Input: part model. Units: mm. Frame: model coordinates. Face numbers are marked on the shaded views. Round coordinates to 2 decimals unless told otherwise and drop trailing zeros. Loops run counter-clockwise (first coordinate to the right, second up) from the corner with the lowest first, then second, coordinate; pieces in that order, holes last. Notation, with made-up numbers: (71, -11) - (84, -11) arc R17 cw to (84, 1) - close; hole circle Ø11 at (-27.5, -19.75). An arc over 180 degrees is marked (long way). One line per question, with ' | ' between items. Start each with the question number.
Item 1: Section B-B, the plane x = 22. Return loops of the section in (y, z), plus the area to 3 significant figures.
Item 2: Section D-D, the plane y = 30.5. Return loops of the section in (x, z), plus the area to 3 significant figures.
Item 3: Material intervals for line 1 along Y through (x, z) = (20, -15); line 2 along X through (y, z) = (31.5, -15); line 3 along Y through (x, z) = (21.5, -42), sorted ascending.
Item 4: First-contact query: pin 1 (12 mm diameter, centred on x = 11, z = -30.5, fed in from -Y); pin 2 (1.3 mm diameter, centred on x = 13.5, z = -23, fed in from +Y); pin 3 (3 mm diameter, centred on x = 1.5, y = 9.5, fed in from -Z); pin 4 (10 mm diameter, centred on y = 4, z = -32.5, fed in from -X). Flat tips, straight axial feed; report the tip coordinate or a pass-through.
Item 5: Section A-A, the plane z = -22. Return loops of the section in (x, y), plus the area to 3 significant figures.
Item 6: Draft query along Y for the marked faces 1, 2 and 3. Return one class per face: pulls with the +Y half, pulls with the -Y half, needs draft (parallel to the pull), parting line crosses it, or undercut.
Item 7: Section C-C, the plane z = -5.5. Return loops of the section in (x, y).
```python
from build123d import *

# Parameters (mm, degrees)
BOSS_EXTRUDE1_DEPTH      = 2.54
BOSS_EXTRUDE2_DEPTH      = 2.54
BOSS_EXTRUDE2_DEPTH_BACK = 12.7
SKETCH3_R                = 1.778
SKETCH4_R                = 34.29
BOSS_EXTRUDE3_DEPTH      = 10.16
BOSS_EXTRUDE4_DEPTH      = 2.54
BOSS_EXTRUDE5_DEPTH      = 10.16
BOSS_EXTRUDE5_DEPTH_BACK = 5.08
SKETCH6_R                = 1.778
SKETCH7_R                = 33.02
CUT_EXTRUDE1_DEPTH       = 7.62
SKETCH9_R                = 2.54
BOSS_EXTRUDE6_DEPTH      = 1.27
SKETCH10_R               = 1.27
BOSS_EXTRUDE7_DEPTH      = 20.32
CUT_EXTRUDE2_REACH       = 65.993
CUT_EXTRUDE3_REACH       = 65.993


with BuildPart() as part:
    # Sketch2 → Boss-Extrude1 (new body)
    with BuildSketch(Plane(origin=(0, 0, 0), x_dir=(0, 0, -1), z_dir=(1, 0, 0))):
        with BuildLine():
            Line((0, -1.778), (30.48, -1.778))
            ThreePointArc((30.48, -1.778), (32.258, 0), (30.48, 1.778))
            Line((30.48, 1.778), (0, 1.778))
            ThreePointArc((0, 1.778), (-1.778, 0), (0, -1.778))
        make_face()
    extrude(amount=BOSS_EXTRUDE1_DEPTH)

    # Sketch3 → Boss-Extrude2 (add, two sides: drawn at the far end of the back side and taken through both)
    with BuildSketch(Plane.ZY.offset(-BOSS_EXTRUDE2_DEPTH_BACK)):
        with Locations((-30.48, 0)):
            Circle(SKETCH3_R)
        Circle(SKETCH3_R)
    extrude(amount=BOSS_EXTRUDE2_DEPTH + BOSS_EXTRUDE2_DEPTH_BACK)

    # Sketch4 → Boss-Extrude3 (add)
    with BuildSketch(Plane(origin=(12.7, 0, 0), x_dir=(0, 0, -1), z_dir=(1, 0, 0))):
        with Locations((15.24, 0)):
            Circle(SKETCH4_R)
    extrude(amount=BOSS_EXTRUDE3_DEPTH)

    # Sketch5 → Boss-Extrude4 (add)
    with BuildSketch(Plane(origin=(0, 0, 0), x_dir=(0, 0, -1), z_dir=(1, 0, 0))):
        with BuildLine():
            Line((13.462, -19.05), (13.462, 19.05))
            ThreePointArc((13.462, 19.05), (15.24, 20.828), (17.018, 19.05))
            Line((17.018, 19.05), (17.018, -19.05))
            ThreePointArc((17.018, -19.05), (15.24, -20.828), (13.462, -19.05))
        make_face()
    extrude(amount=BOSS_EXTRUDE4_DEPTH)

    # Sketch6 → Boss-Extrude5 (add, two sides: drawn at the far end of the back side and taken through both)
    with BuildSketch(Plane(origin=(2.54, 0, 0), x_dir=(0, 0, -1), z_dir=(1, 0, 0)).offset(-BOSS_EXTRUDE5_DEPTH_BACK)):
        with Locations((15.24, -19.05)):
            Circle(SKETCH6_R)
        with Locations((15.24, 19.05)):
            Circle(SKETCH6_R)
    extrude(amount=BOSS_EXTRUDE5_DEPTH + BOSS_EXTRUDE5_DEPTH_BACK)

    # Sketch7 → Cut-Extrude1 (cut)
    with BuildSketch(Plane(origin=(22.86, 0, 0), x_dir=(0, 0, -1), z_dir=(1, 0, 0))):
        with Locations((15.24, 0)):
            Circle(SKETCH7_R)
    extrude(amount=-CUT_EXTRUDE1_DEPTH, mode=Mode.SUBTRACT)

    # Sketch9 → Boss-Extrude6 (add)
    with BuildSketch(Plane(origin=(15.24, 0, 0), x_dir=(0, 0, -1), z_dir=(1, 0, 0))):
        Circle(SKETCH9_R)
        with Locations((30.48, 0)):
            Circle(SKETCH9_R)
    extrude(amount=BOSS_EXTRUDE6_DEPTH)

    # Sketch10 → Boss-Extrude7 (add)
    with BuildSketch(Plane(origin=(16.51, 0, 0), x_dir=(0, 0, -1), z_dir=(1, 0, 0))):
        with Locations((30.48, 0)):
            Circle(SKETCH10_R)
        Circle(SKETCH10_R)
    extrude(amount=BOSS_EXTRUDE7_DEPTH)

    # Sketch11 → Cut-Extrude2 (cut, up to next)
    with BuildSketch(Plane(origin=(15.24, 0, 0), x_dir=(0, 0, -1), z_dir=(1, 0, 0)), mode=Mode.PRIVATE) as cut_extrude2_sk1:
        with BuildLine():
            Line((14.51, 5), (15.97, 5))
            ThreePointArc((15.97, 5), (16.868025612, 4.628025612), (17.24, 3.73))
            Line((17.24, 3.73), (17.24, -3.73))
            ThreePointArc((17.24, -3.73), (16.868025612, -4.628025612), (15.97, -5))
            Line((15.97, -5), (14.51, -5))
            ThreePointArc((14.51, -5), (13.611974388, -4.628025612), (13.24, -3.73))
            Line((13.24, -3.73), (13.24, 3.73))
            ThreePointArc((13.24, 3.73), (13.611974388, 4.628025612), (14.51, 5))
        make_face()
    cut_extrude2_tool1 = extrude(cut_extrude2_sk1.sketch, amount=-CUT_EXTRUDE2_REACH, mode=Mode.PRIVATE) & part.part
    add(cut_extrude2_tool1.solids().sort_by_distance((15.24, 0, -15.24))[0], mode=Mode.SUBTRACT)

    # Sketch15 → Cut-Extrude3 (cut, up to next)
    with BuildSketch(Plane(origin=(15.24, 0, 0), x_dir=(0, 0, -1), z_dir=(1, 0, 0)), mode=Mode.PRIVATE) as cut_extrude3_sk1:
        with BuildLine():
            Line((16.51, 10), (33.97, 10))
            ThreePointArc((33.97, 10), (34.868025612, 10.371974388), (35.24, 11.27))
            Line((35.24, 11.27), (35.24, 13.73))
            ThreePointArc((35.24, 13.73), (34.868025612, 14.628025612), (33.97, 15))
            Line((33.97, 15), (16.51, 15))
            ThreePointArc((16.51, 15), (15.611974388, 14.628025612), (15.24, 13.73))
            Line((15.24, 13.73), (15.24, 11.27))
            ThreePointArc((15.24, 11.27), (15.611974388, 10.371974388), (16.51, 10))
        make_face()
    cut_extrude3_tool1 = extrude(cut_extrude3_sk1.sketch, amount=-CUT_EXTRUDE3_REACH, mode=Mode.PRIVATE) & part.part
    add(cut_extrude3_tool1.solids().sort_by_distance((15.24, 12.5, -25.24))[0], mode=Mode.SUBTRACT)


solid = part.part
```
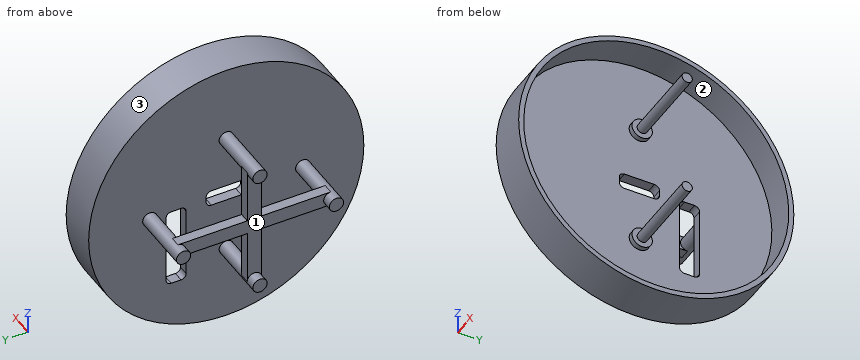
Return value:
1) outline: circle Ø68.58 at (0, -15.24); circle Ø2.54 at (0, -30.48); circle Ø2.54 at (0, 0); hole circle Ø66.04 at (0, -15.24) | area: 279 mm2
2) outline: (12.7, -30.91) - (22.86, -30.91) - (22.86, -27.89) - (15.24, -27.89) - (15.24, -2.59) - (22.86, -2.59) - (22.86, 0.43) - (12.7, 0.43) - close | area: 126 mm2
3) line 1: -34.29 to -33.02, 33.02 to 34.29 | line 2: 12.7 to 15.24 | line 3: -21.44 to -19.34, 19.34 to 21.44
4) pin 1: y = -32.95 | pin 2: y = 33.54 | pin 3: z = -17.02 | pin 4: x = -2.54
5) outline: (0, -1.78) - (2.54, -1.78) - (2.54, 1.78) - (0, 1.78) - close; (12.7, -33.62) - (22.86, -33.62) - (22.86, -32.32) - (15.24, -32.32) - (15.24, 10) - (12.7, 10) - close; (12.7, 15) - (15.24, 15) - (15.24, 32.32) - (22.86, 32.32) - (22.86, 33.62) - (12.7, 33.62) - close | area: 187 mm2
6) face 1: undercut | face 2: undercut | face 3: parting line crosses it
7) outline: (0, -1.78) - (2.54, -1.78) - (2.54, 1.78) - (0, 1.78) - close; (12.7, -32.88) - (22.86, -32.88) - (22.86, -31.55) - (15.24, -31.55) - (15.24, 31.55) - (22.86, 31.55) - (22.86, 32.88) - (12.7, 32.88) - close
